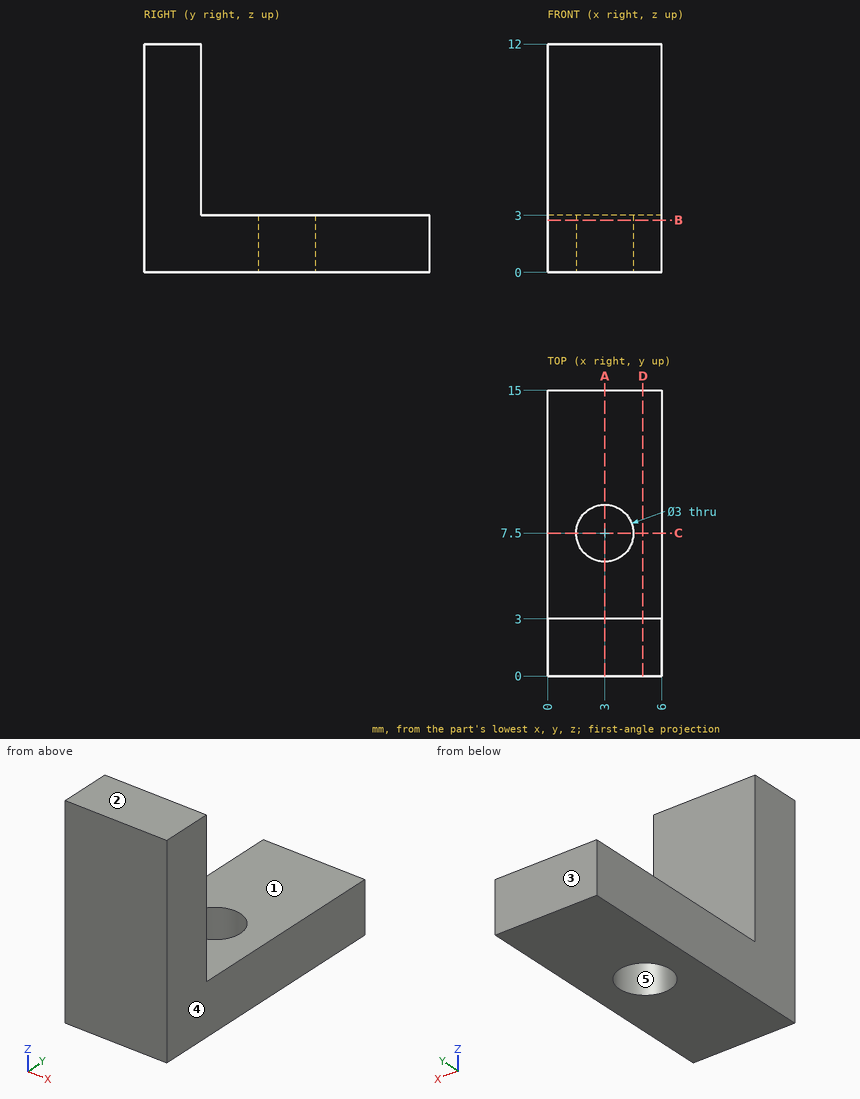
Part print with two shaded views. Sizes in mm from the minimum x, y, z corner. A direction names the side the tool comes from. Coordinates: 2 decimals unless noted, no trailing zeros. Write each loop counter-clockwise with the first axis right and the second up, starting at its lowest first coordinate (ties: lowest second). Pieces come first, ordered by that corner, then holes. Notation, with made-up numbers: (2.5, 69.25) - (6.5, 69.25) arc R21 cw to (6.5, 100.25) - close; hole circle Ø3 at (-33, -16). An arc over 180 degrees is marked (long way). One line per item, written item: value. Start each with the question number.
1. Tool access for the marked faces 1 and 2: list every direction of +Z, -Z, +X, -X, +Y, -Y with a clear straight run to the whole face (end or side of a thin tool).
2. Slice it at C-C (y = 7.5). Write the cut outline in (x, z).
3. Probe line 1 (Y direction, x = 3, z = 1.3); line 2 (Z direction, x = 4.2, y = 12); line 3 (X direction, y = 7.5, z = 2.2). List the from-to ranges inside material, lowest first. Write a range as from..to.
4. Mould opens along X. For the marked faces 3, 4 and 5 say: released by +X, released by -X, zero draft, split by the parting line, or undercut.
5. Slice it at D-D (x = 5). Write the cut outline in (y, z).
6. Slice it at B-B (z = 2.75). Write the cut outline in (x, y), plus the area to 3 significant figures.
7. Flat gauge pins, fed straight in: pin 1 (3.5 mm diameter, centred on x = 3, y = 7.5, fed in from +Z); pin 2 (1.8 mm diameter, centred on x = 2, z = 9, fed in from +Y). Where does each tip first touch, or does it go through?
8. Slice it at A-A (x = 3). Write the cut outline in (y, z), plus the area to 3 significant figures.
Answers below:
1. face 1: +Z, +X, -X, +Y
1. face 2: +Z, +X, -X, +Y, -Y
2. outline: (0, 0) - (1.5, 0) - (1.5, 3) - (0, 3) - close; (4.5, 0) - (6, 0) - (6, 3) - (4.5, 3) - close
3. line 1: y = 0..6, 9..15
3. line 2: z = 0..3
3. line 3: x = 0..1.5, 4.5..6
4. face 3: zero draft
4. face 4: released by +X
4. face 5: undercut
5. outline: (0, 0) - (15, 0) - (15, 3) - (3, 3) - (3, 12) - (0, 12) - close
6. outline: (0, 0) - (6, 0) - (6, 15) - (0, 15) - close; hole circle Ø3 at (3, 7.5)
6. area: 82.9 mm^2
7. pin 1: stops at z = 3
7. pin 2: stops at y = 3
8. outline: (0, 0) - (6, 0) - (6, 3) - (3, 3) - (3, 12) - (0, 12) - close; (9, 0) - (15, 0) - (15, 3) - (9, 3) - close
8. area: 63.0 mm^2
